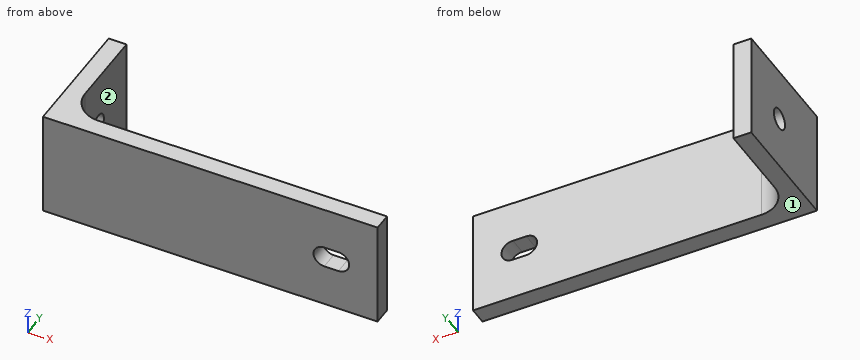
```python
from build123d import *

# Parameters (mm, degrees)
F1_DEPTH = 15
F3_D     = 2.95
F4_R     = 4
F6_DEPTH = 25


with BuildPart() as f1:
    # F0 (on Top) → F1 (new body)
    with BuildSketch(Plane.XY):
        Polygon((44.5, 0), (0, 0), (0, 15), (-2.5, 15), (-2.5, -2.5), (44.5, -2.5), align=None)
    extrude(amount=F1_DEPTH)

    # F3 (through all)
    with Locations(Plane.YZ):
        with Locations((7.5, 7.5)):
            Hole(F3_D / 2)

    # F4
    f4_edges = [f1.edges().sort_by_distance(p)[0] for p in [
        (0, 0, 7.5),
    ]]
    fillet(f4_edges, radius=F4_R)

    # F5 (on face) → F6 (cut)
    with BuildSketch(Plane(origin=(0, 0, 0), x_dir=(-1, 0, 0), z_dir=(0, 1, 0))):
        with BuildLine():
            Line((-39, 6), (-37, 6))
            ThreePointArc((-37, 6), (-35.500001, 7.501758), (-37.003516, 8.999996))
            Line((-37.003516, 8.999996), (-38.88501, 8.995586))
            ThreePointArc((-38.88501, 8.995586), (-40.498896, 7.557537), (-39, 6))
        make_face()
    extrude(amount=-F6_DEPTH, mode=Mode.SUBTRACT)


solid = f1.part
```
Build history of the part. All positions in model axes, mm. Face numbers are marked on the shaded views. A direction names the side the tool comes from. Round coordinates to 2 decimals unless told otherwise and drop trailing zeros. Loops run counter-clockwise (first coordinate to the right, second up) from the corner with the lowest first, then second, coordinate; pieces in that order, holes last. Notation, with made-up numbers: M 26,5.5 L 53,5.5 A10 cw 53,17.5 Z; hole C -3.5,69.5 d9. An arc over 180 degrees is marked long. Answer as CSV lines item,"result".
1. Wall check: probe 1 along Z at (x, y) = (-0.85, 7.5) (3 decimals); probe 2 along X at (y, z) = (8.5, 10). Give the ranges that are in metal, low to high. Write a range as [from, to].
Resolved:
probe 1,"z = [0, 6.025], [8.975, 15]"
probe 2,"x = [-2.5, 0]"
2. Cut at C-C on z = 13. Write the cut outline in (x, y), then the cut area to 3 significant figures.
Resolved:
outline,"M -2.5,-2.5 L 44.5,-2.5 L 44.5,0 L 4,0 A4 cw 0,4 L 0,15 L -2.5,15 Z"
area,"158 mm²"
3. Cut at A-A on y = 7.5. Write the cut outline in (x, z) (3 decimals).
Resolved:
outline,"M -2.5,0 L 0,0 L 0,6.025 L -2.5,6.025 Z; M -2.5,8.975 L 0,8.975 L 0,15 L -2.5,15 Z"
4. Flat gauge pins, fed straight in: P1, Ø1, axis at x = 26.5, z = 2.5, coming from the +Y side; P2, Ø2.5, axis at y = 7.5, z = 7.5, coming from the -X side; P3, Ø6, axis at y = 10.5, z = 3, coming from the +X side. Where does each tip first touch, or does it go through?
Resolved:
P1,"stops at y = 0"
P2,"passes through"
P3,"stops at x = 0"
5. Cut at B-B on z = 7.5. Write the cut outline in (x, y) (3 decimals).
Resolved:
outline,"M -2.5,-2.5 L 35.5,-2.5 L 35.5,0 L 4,0 A4 cw 0,4 L 0,6.025 L -2.5,6.025 Z; M -2.5,8.975 L 0,8.975 L 0,15 L -2.5,15 Z; M 40.5,-2.5 L 44.5,-2.5 L 44.5,0 L 40.5,0 Z"
6. 3-axis set-ups, long thin cutter, end or side, ignore diameter. For the marked faces 1 and 2: which of +Z, -Z, +X, -X, +Y, -Y reach the whole face in a straight line?
Resolved:
face 1,"-Z, +X, -X, +Y, -Y"
face 2,"+Z, -Z, +X, +Y"
7. Cut at D-D on x = 11. Write the cut outline in (y, z), then the cut area to 3 significant figures.
Resolved:
outline,"M -2.5,0 L 0,0 L 0,15 L -2.5,15 Z"
area,"37.5 mm²"
